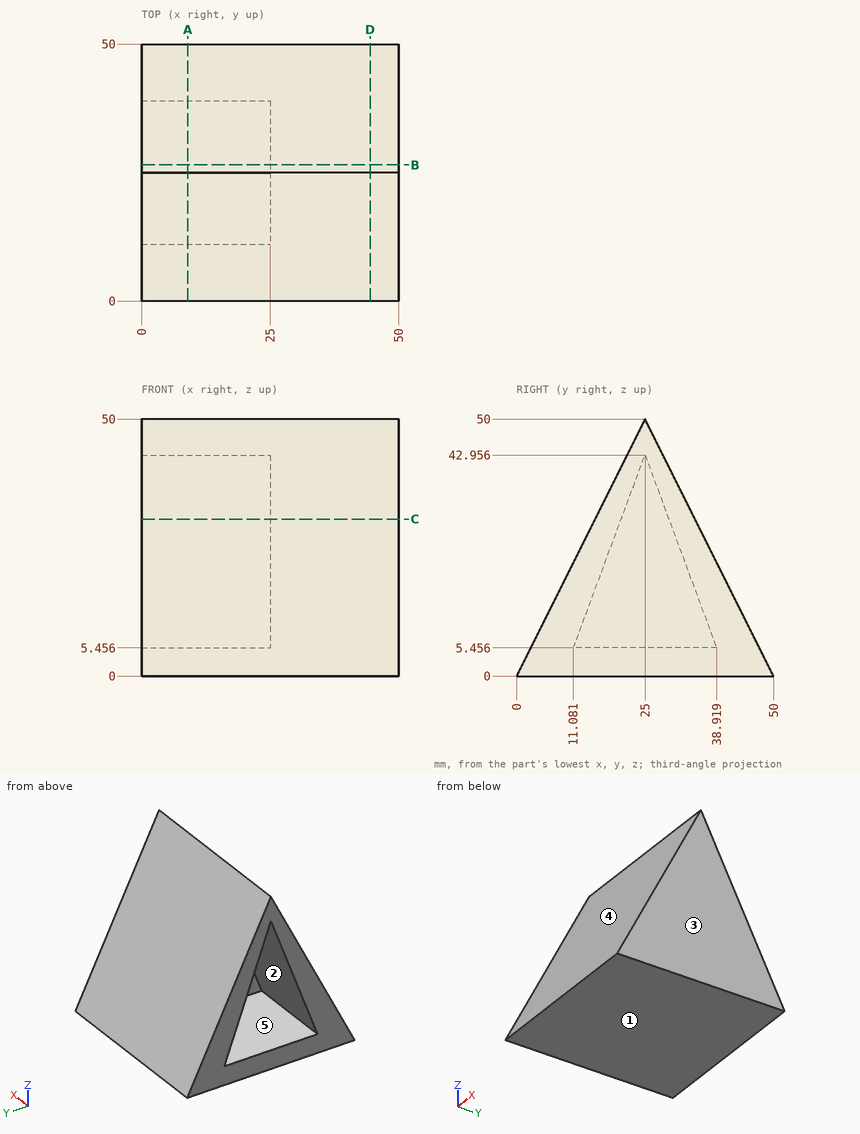
The figure shows three views and two pictorial views of one solid part (mm, origin at its lowest corner). Answer the questions. A direction names the side the tool comes from. Round coordinates to 2 decimals unless told otherwise and drop trailing zeros. Order: outer loops, then holes, each group sorted by start corner. A loop starts at its lowest first (then second) coordinate and runs counter-clockwise, first axis right, second up. Notation, with made-up numbers: M 89,82.5 L 141,82.5 A6 cw 141,90.5 Z; hole C -34,57 d11. An arc over 180 degrees is marked long. Answer in a Markdown table with one row per item. Add a question column.
1) The part is cut by section B-B on y = 26.5. Determine the outline of the cut face in (x, z) (1 decimal), plus the area to 3 significant figures.
2) The part is cut by section D-D on x = 44.5. Determine the outline of the cut face in (y, z), plus the area to 3 significant figures.
3) Flat-ended cylindrical pins translate along their axes: pin 1 Ø2 at (x, z) = (41, 26.5) entering from +Y; pin 2 Ø1.5 at (x, z) = (29, 43) entering from -Y (1 decimal); pin 3 Ø3 at (y, z) = (16, 37) entering from +X; pin 4 Ø10 at (x, z) = (25, 15.5) entering from +Y. Find the tip coordinate at first contact, or state that the pin passes through.
4) The part is cut by section A-A on x = 9. Determine the outline of the cut face in (y, z), plus the area to 3 significant figures.
5) Which of the six approach directions +Z, -Z, +X, -X, +Y, -Y give full straight-line access (tool end or side, diameter ignored) to the marked faces 4 and 5?
6) The part is cut by section C-C on z = 30.5. Determine the outline of the cut face in (x, y).
7) Determine the mould class of the marked faces 1, 2 and 3 for opening direction Z: pulls with the +Z half, pulls with the -Z half, needs draft (parallel to the pull), parting line crosses it, or undercut.
8) Consider line 1 along Y through (x, z) = (2, 22.5); line 2 along X through (y, z) = (28, 24); line 3 along Y through (x, z) = (17, 30). Determine where each line is inside the solid, lowest interval first. Write a range as from..to.
Findings below:
| question | item | result |
|---|---|---|
| 1 | outline | M 0,0 L 50,0 L 50,47 L 0,47 L 0,38.9 L 25,38.9 L 25,5.5 L 0,5.5 Z |
| 1 | area | 1,510 mm² |
| 2 | outline | M 0,0 L 50,0 L 25,50 Z |
| 2 | area | 1,250 mm² |
| 3 | pin 1 | stops at y = 37.25 |
| 3 | pin 2 | stops at y = 21.1 |
| 3 | pin 3 | passes through |
| 3 | pin 4 | stops at y = 44.75 |
| 4 | outline | M 0,0 L 50,0 L 25,50 Z; hole M 11.08,5.46 L 38.92,5.46 L 25,42.96 Z |
| 4 | area | 728 mm² |
| 5 | face 4 | +Z, +X, -X, -Y |
| 5 | face 5 | -X |
| 6 | outline | M 0,15.25 L 50,15.25 L 50,34.75 L 0,34.75 L 0,29.62 L 25,29.62 L 25,20.38 L 0,20.38 Z |
| 7 | face 1 | pulls with the -Z half |
| 7 | face 2 | undercut |
| 7 | face 3 | needs draft |
| 8 | line 1 | y = 11.25..17.41, 32.59..38.75 |
| 8 | line 2 | x = 25..50 |
| 8 | line 3 | y = 15..20.19, 29.81..35 |
